from build123d import *

# Parameters (mm, degrees)
F1_DEPTH = 101.6
F3_DEPTH = 130.048
F4_W     = 11.070052
F4_H     = 38.1
F5_DEPTH = 60.198


with BuildPart() as f1:
    # F0 (on Right) → F1 (new body)
    with BuildSketch(Plane.YZ):
        Polygon((11.070052, 44.179608), (-27.029948, 44.179608), (-27.029948, -6.620392), (-52.429948, -6.620392), (-52.429948, -32.020392), (11.070052, -32.020392), align=None)
    extrude(amount=F1_DEPTH)

    # F2 (on face) → F3 (cut)
    with BuildSketch(Plane.XZ.offset(27.029948)):
        Polygon((76.2, 44.179608), (50.8, 44.179608), (25.4, 44.179608), (25.4, 6.079608), (76.2, 6.079608), align=None)
    extrude(amount=-F3_DEPTH, mode=Mode.SUBTRACT)

    # F4 (on face) → F5 (join)
    with BuildSketch(Plane(origin=(76.2, 0, 0), x_dir=(0, -1, 0), z_dir=(-1, 0, 0))):
        with Locations((-5.535026, 25.129608)):
            Rectangle(F4_W, F4_H)
    extrude(amount=F5_DEPTH)


solid = f1.part
Could you check a few things on this model? Use its own coordinates, in mm. A direction names the side the tool comes from. Coordinates: 2 decimals unless noted, no trailing zeros. Loops run counter-clockwise (first coordinate to the right, second up) from the corner with the lowest first, then second, coordinate; pieces in that order, holes last.
1. For faces 1 (the face through (50, -21, -32.02)), 2 (the face through (50, -27.03, 2)), 3 (the face through (50, -14, 6.08)), which set-ups out of +Z, -Z, +X, -X, +Y, -Y let a thin tool reach every point of the face, with its end or its side?
2. We'd pull the mould along X, two halves only. Please class faces 4 (the face through (50, 1, 44.18)), 5 (the face through (0, -14, -2)), 6 (the face through (51, 0, 25)), 7 (the face through (101.6, -14, -2)): released by +X, released by -X, zero draft, split by the parting line, or undercut.
3. Imagine slicing it at C-C (y = -29). Please give me the cut outline in (x, z).
4. Imagine slicing it at A-A (x = 33). Please give me the cut outline in (y, z), and give its area (3 significant figures).
5. Imagine slicing it at D-D (x = 12). Please give me the cut outline in (y, z).
6. For P1, Ø20.5, axis at x = 52.5, y = -37, coming from the +Z side; P2, Ø11.5, axis at x = 63, z = 33, coming from the -Y side; P3, Ø4, axis at y = 1.5, z = -22.5, coming from the -X side; P4, Ø2, axis at x = 14.5, y = -34, coming from the +Z side, each with a flat end and sliding along its axis, tell me the tip position at first contact or that it passes through.
7. I need wall thicknesses on L1, parallel to X at y = -11.5, z = 21.5; L2, parallel to Z at x = 67, y = -41.5; L3, parallel to Y at x = 46.5, z = 20. Which ranges of each line are inside material? Lowest first, please.
8. Imagine slicing it at B-B (z = 8). Please give me the cut outline in (x, y), and give its area (3 significant figures).
Computed values:
1. face 1: -Z, +X, -X, +Y, -Y
1. face 2: +Z, +X, -X, -Y
1. face 3: +Z, -Y
2. face 4: zero draft
2. face 5: released by -X
2. face 6: undercut
2. face 7: released by +X
3. outline: (0, -32.02) - (101.6, -32.02) - (101.6, -6.62) - (0, -6.62) - close
4. outline: (-52.43, -32.02) - (11.07, -32.02) - (11.07, 44.18) - (0, 44.18) - (0, 6.08) - (-27.03, 6.08) - (-27.03, -6.62) - (-52.43, -6.62) - close
4. area: 2,520 mm2
5. outline: (-52.43, -32.02) - (11.07, -32.02) - (11.07, 44.18) - (-27.03, 44.18) - (-27.03, -6.62) - (-52.43, -6.62) - close
6. P1: stops at z = 6.08
6. P2: stops at y = 0
6. P3: stops at x = 0
6. P4: stops at z = -6.62
7. L1: x = 0 to 25.4, 76.2 to 101.6
7. L2: z = -32.02 to -6.62
7. L3: y = 0 to 11.07
8. outline: (0, -27.03) - (25.4, -27.03) - (25.4, 0) - (76.2, 0) - (76.2, -27.03) - (101.6, -27.03) - (101.6, 11.07) - (0, 11.07) - close
8. area: 2,500 mm2
